Source: CAD feature listing. Evaluate the final solid. Frame: model axes, mm. A direction names the side the tool comes from. Coordinates: 2 decimals unless noted, no trailing zeros. Loops run counter-clockwise (first coordinate to the right, second up) from the corner with the lowest first, then second, coordinate; pieces in that order, holes last. Notation, with made-up numbers: (-21, 16) - (-5, 16) arc R13 ccw to (-5, 27) - close; hole circle Ø9 at (32.5, 8). An arc over 180 degrees is marked (long way). Write item = value, one per line. Start each with the question number.
from build123d import *

# Parameters (mm, degrees)
SKETCH1_W           = 114.3
SKETCH1_H           = 63.5
BOSS_EXTRUDE1_DEPTH = 3.175
BOSS_EXTRUDE2_DEPTH = 3.175
BOSS_EXTRUDE3_START = -57.15
BOSS_EXTRUDE3_DEPTH = 114.3
CUT_EXTRUDE1_DEPTH  = 125.91911954
CHAMFER1_SIZE       = 2.54


# Read off the part's stored shape, not the designer's step: Boss-Extrude3
with BuildPart() as part:
    # Sketch1 → Boss-Extrude1 (new body)
    with BuildSketch(Plane(origin=(0, 0, 0), x_dir=(1, 0, 0), z_dir=(0, 1, 0))):
        Rectangle(SKETCH1_W, SKETCH1_H)
    extrude(amount=BOSS_EXTRUDE1_DEPTH)

    # Sketch2 → Boss-Extrude2 (add)
    with BuildSketch(Plane(origin=(0, 0, -31.75), x_dir=(-1, 0, 0), z_dir=(0, 0, -1))):
        Polygon((-16.15831866, 36.339246026), (39.380032744, 5.55383514), (36.301491655, 0), (-36.301491655, 0), align=None)
    extrude(amount=BOSS_EXTRUDE2_DEPTH)

    # Boss-Extrude3 outline → Boss-Extrude3 (add)
    with BuildSketch(Plane.YZ.offset(BOSS_EXTRUDE3_START)):
        Polygon((14.371763275, 31.75), (3.175, 31.75), (3.175, -31.75), align=None)
    extrude(amount=BOSS_EXTRUDE3_DEPTH)

    # Sketch4 → Cut-Extrude1 (cut, through all)
    with BuildSketch(Plane(origin=(57.15, 0, 0), x_dir=(0, 0, -1), z_dir=(1, 0, 0))):
        Polygon((-31.75, 12.3084164), (-31.75, 0), (34.925, 0), (34.925, 0.551814961), align=None)
    extrude(amount=-CUT_EXTRUDE1_DEPTH, mode=Mode.SUBTRACT)

    # Chamfer1
    # the kernel refuses this chamfer: 2.54 mm, written as the material it adds along each edge
    with BuildSketch(Plane(origin=(-45.794774456, 3.175, -31.75), x_dir=(0, 0.14881491150796153, 0.988865067697751), z_dir=(1, 0, 0))) as chamfer1_piece_1_section:
        Polygon((CHAMFER1_SIZE * 1.19137631147, -CHAMFER1_SIZE * 0.0299851619673), (CHAMFER1_SIZE * 0.177350705421, -CHAMFER1_SIZE * 1.17848349702), (0, 0), align=None)
    chamfer1_piece_1 = extrude(amount=88.069686436, mode=Mode.PRIVATE)
    chamfer1_piece_1 = split(chamfer1_piece_1, bisect_by=Plane(origin=(-30.181920022, -11.039999469, -30.75599928), z_dir=(0.8746197071393951, 0.48480962024633845, 0)), keep=Keep.TOP, mode=Mode.PRIVATE)
    chamfer1_piece_1 = split(chamfer1_piece_1, bisect_by=Plane(origin=(25.356431382, 19.745411417, -30.75599928), z_dir=(-0.8746197071393954, -0.4848096202463377, 0)), keep=Keep.TOP, mode=Mode.PRIVATE)
    chamfer1_piece_1 = split(chamfer1_piece_1, bisect_by=Plane(origin=(-11.60015099, 20.952475045, -30.75599928), z_dir=(0.4848096202463377, -0.8746197071393954, 0)), keep=Keep.TOP, mode=Mode.PRIVATE)
    add(chamfer1_piece_1)


solid = part.part
Item 1: Cut plane D-D (x = -2.5). Return the cut outline in (y, z) (3 decimals), then the cut area to 3 significant figures.
Item 2: Cut plane B-B (x = -20.5). Return the cut outline in (y, z) (3 decimals), then the cut area to 3 significant figures.
Item 3: Material intervals for L1, parallel to Z at x = 18, y = 24 (3 decimals); L2, parallel to Y at x = 20, z = -11.5; L3, parallel to Y at x = 15, z = -31, sorted ascending. Write a range as [from, to].
Item 4: Cut plane A-A (y = 8). Return the cut outline in (x, z) (3 decimals).
Item 5: Reachability of faces 5 (the flat face through (5, 15, -31.75)), 6 (the flat face through (57.15, 8, 0)) from +Z, -Z, +X, -X, +Y, -Y: full face, straight path, thin tool, end or side. Return the list, or none.
Item 6: Draft query along Z for faces 1 (the flat face through (-3.1, 4.9, -30.2)), 2 (the flat face through (-11.222, 21.162, -33.417)), 3 (the flat face through (-1, 13, 31.75)), 4 (the flat face through (46, 2, -31.75)). Return one class per face: released by +Z, released by -Z, zero draft, split by the parting line, or undercut.
Item 7: First-contact query: pin 1 (4 mm diameter, centred on x = -42, y = 17, fed in from +Z); pin 2 (0.6 mm diameter, centred on x = -49.5, y = 1.5, fed in from -Z); pin 3 (1 mm diameter, centred on x = 39, z = -16, fed in from -Y); pin 4 (6 mm diameter, centred on x = 39.5, z = 15.5, fed in from -Y). Flat tips, straight axial feed; report the tip coordinate or a pass-through.
Item 8: Cut plane C-C (z = 10.5). Return the cut outline in (x, y), then the cut area to 3 significant figures.
Responses:
q1.outline = (0.552, -34.925) - (25.997, -34.925) - (25.997, -31.75) - (6.202, -31.75) - (3.701, -28.769) - (14.372, 31.75) - (12.308, 31.75) - close
q1.area = 215 mm2
q2.outline = (0.552, -34.925) - (16.019, -34.925) - (16.019, -31.75) - (6.202, -31.75) - (3.701, -28.769) - (14.372, 31.75) - (12.308, 31.75) - close
q2.area = 184 mm2
q3.L1 = [-34.925, -31.75]
q3.L2 = [4.68, 6.75]
q3.L3 = [1.24, 5.57]
q4.outline = (-57.15, -4.386) - (57.15, -4.386) - (57.15, 7.316) - (-57.15, 7.316) - close; (-34.967, -34.925) - (31.867, -34.925) - (31.867, -31.75) - (-34.967, -31.75) - close
q5.face_5 = +X, -X, +Y
q5.face_6 = +Z, -Z, +X, +Y, -Y
q6.face_1 = undercut
q6.face_2 = zero draft
q6.face_3 = released by +Z
q6.face_4 = released by -Z
q7.pin_1 = through
q7.pin_2 = -31.75
q7.pin_3 = 3.8
q7.pin_4 = 8.91
q8.outline = (-57.15, 8.56) - (57.15, 8.56) - (57.15, 10.62) - (-57.15, 10.62) - close
q8.area = 236 mm2
